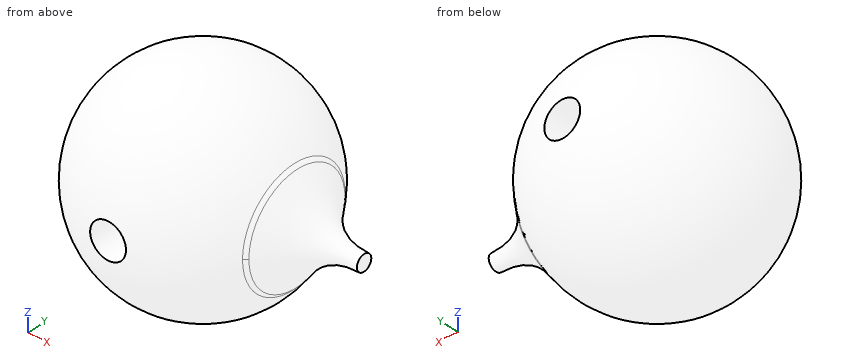
```python
from build123d import *

# Parameters (mm, degrees)
F3_R        = 10.16
F4_DEPTH    = 15.875
F7_R        = 3.175
F8_DEPTH    = 25.4
F9_T2_ANGLE = 180.0000002199
F9_T4_ANGLE = 179.9999999345


# Not quite as in the source:
# - a fillet or chamfer that OpenCascade refuses, or shapes differently, is made with other operations: its cross-section is extruded or revolved along the edge and cut away or added


with BuildPart() as f1:
    # F0 (on Front) → F1 (revolve)
    with BuildSketch(Plane.XZ):
        with BuildLine():
            Line((0, 19.05), (0, -19.05))
            ThreePointArc((0, -19.05), (19.05, 0), (0, 19.05))
        make_face()
    revolve(axis=Axis((0, 0, 0), (0, 0, -1)))

    # F3 (on offset) → F4 (join)
    with BuildSketch(Plane.YZ.offset(12.7)):
        Circle(F3_R)
    extrude(amount=F4_DEPTH)

    # F5 (on Top) → F6 (revolve, cut)
    with BuildSketch(Plane.XY):
        with BuildLine():
            add(Edge.make_bspline(
                [(16.0334594548, -10.3644961491), (17.5619016312, -8.4434705035), (22.291404173, -0.7556150252), (28.8937536319, -1.4395783264), (30.1896631718, -1.4926075237)],
                knots=[0, 0, 0, 0, 0.5565187358, 1, 1, 1, 1], degree=3))
            Line((16.0334594548, -10.3644961491), (30.1896631718, -10.3644961491))
            Line((30.1896631718, -10.3644961491), (30.1896631718, -1.4926075237))
        make_face()
    revolve(axis=Axis((23.3597867191, 0, 0), (-1, 0, 0)), mode=Mode.SUBTRACT)

    # F7 (on Front) → F8 (cut, symmetric)
    with BuildSketch(Plane.XZ):
        Circle(F7_R)
    extrude(amount=F8_DEPTH, both=True, mode=Mode.SUBTRACT)

    # F9: fillet of radius 5.08 on 2 edges, made by hand

    # F9_s1 → F9_t2 (revolve, cut)
    with BuildSketch(Plane.XY.offset(-1.95e-08)):
        with BuildLine():
            ThreePointArc((16.1144934764, -10.1599999963), (16.407046723, -9.8527346061), (16.6729403711, -9.5221291161))
            Line((16.6729403711, -9.5221291161), (16.7547016298, -9.5824421047))
            ThreePointArc((16.7547016298, -9.5824421047), (16.5162775071, -9.9033020934), (16.2740232311, -10.2220962285))
            Line((16.2740232311, -10.2220962285), (16.1936079439, -10.2616))
            ThreePointArc((16.1936079439, -10.2616), (16.1540507101, -10.2615999963), (16.1850857971, -10.2330704024))
            Line((16.1850857971, -10.2330704024), (16.1144934764, -10.1599999963))
        make_face()
    revolve(axis=Axis((16.1936079439, -1.58e-08, -1.95e-08), (1, 0, 0)), revolution_arc=F9_T2_ANGLE, mode=Mode.SUBTRACT)

    # F9_s3 → F9_t4 (revolve, cut)
    with BuildSketch(Plane.XY.offset(-5.8e-09)):
        with BuildLine():
            ThreePointArc((16.1144934764, 10.1600000025), (16.407046723, 9.8527346123), (16.6729403711, 9.5221291223))
            Line((16.6729403711, 9.5221291223), (16.7547016298, 9.5824421109))
            ThreePointArc((16.7547016298, 9.5824421109), (16.5162775086, 9.9033020976), (16.2740232311, 10.2220962285))
            Line((16.2740232311, 10.2220962285), (16.1936079439, 10.2616))
            ThreePointArc((16.1936079439, 10.2616), (16.1540507101, 10.2616000025), (16.1850857971, 10.2330704086))
            Line((16.1850857971, 10.2330704086), (16.1144934764, 10.1600000025))
        make_face()
    revolve(axis=Axis((16.1936079439, -3.3e-09, -5.8e-09), (1, 0, 0)), revolution_arc=F9_T4_ANGLE, mode=Mode.SUBTRACT)


solid = f1.part
```
Verification items for the finished model (mm, model axes). Round coordinates to 2 decimals unless told otherwise and drop trailing zeros. Write each loop counter-clockwise with the first axis right and the second up, starting at its lowest first coordinate (ties: lowest second). Pieces come first, ordered by that corner, then holes. Notation, with made-up numbers: (56.25, 48) - (93.25, 48) arc R25 cw to (93.25, 65) - close; hole circle Ø6 at (20.25, 8.25). An arc over 180 degrees is marked (long way). Answer as a JSON object with one key per item and string values. Group by question number.
Q1. Section check C-C, the plane z = -15. Enter the section's corners in (x, y), plus the area to 3 significant figures.
Q2. Section check D-D, the plane x = -13.5. Enter the section's corners in (y, z), plus the area to 3 significant figures.
Q3. Thickness scan on line 1 (Z direction, x = 0, y = 0.5) (3 decimals); line 2 (Z direction, x = 0, y = 9) (3 decimals); line 3 (X direction, y = -9, z = 0) (3 decimals). Record the ranges inside material, lowest first.
Q4. Section check A-A, the plane x = 0. Enter the section's corners in (y, z) (3 decimals), plus the area to 3 significant figures.
Q5. Section check B-B, the plane y = 11. Enter the section's corners in (x, z) (3 decimals).
Q6. Go/stop test with flat-tipped pins: pin 1 Ø1.5 at (y, z) = (-8.5, 3) entering from -X; pin 2 Ø6 at (y, z) = (7, -6) entering from -X; pin 3 Ø2 at (x, z) = (16, -0.5) entering from +Y. Record where each tip stops, or that it passes through.
Found:
{
 "1": {"outline": "circle Ø23.49 at (0, 0)", "area": "433 mm^2"},
 "2": {"outline": "circle Ø26.88 at (0, 0)", "area": "568 mm^2"},
 "3": {"line 1": "z = -19.043 to -3.175, 3.175 to 19.043", "line 2": "z = -16.79 to -3.175, 3.175 to 16.79", "line 3": "x = -16.79 to -3.175, 3.175 to 17.056"},
 "4": {"outline": "(-18.784, -3.175) arc R19.05 ccw to (18.784, -3.175) - close; (-18.784, 3.175) - (18.784, 3.175) arc R19.05 ccw to start", "area": "899 mm^2"},
 "5": {"outline": "circle Ø31.106 at (0, 0); hole circle Ø6.35 at (0, 0)"},
 "6": {"pin 1": "stops at x = -17.16", "pin 2": "stops at x = -18.01", "pin 3": "stops at y = 11.73"}
}
